from build123d import *

# Parameters (mm, degrees)
F1_DEPTH = 63.5
F0_W     = 25.4
F0_H     = 4.7498
F0_H_2   = 4.7752
F2_DEPTH = 7.9375


with BuildPart() as f1:
    # F0 (on Front) → F1 (new body, symmetric)
    with BuildSketch(Plane.XZ):
        Polygon((25.4, 9.525), (-44.45, 9.525), (-44.45, -9.525), (44.45, -9.525), (44.45, 9.525), align=None)
    extrude(amount=F1_DEPTH, both=True)

    # F0 (on Front) → F2 (join, symmetric)
    with BuildSketch(Plane.XZ):
        with BuildLine():
            add(Edge.make_bspline(
                [(-44.45, 9.525), (-42.0019178226, 33.4759426415), (20.3692746454, 60.014643523), (58.4090455621, 61.8969537879)],
                knots=[0, 0, 0, 0, 115.3620955336, 115.3620955336, 115.3620955336, 115.3620955336], degree=3))
            Line((-44.45, 9.525), (25.4, 9.525))
            Line((25.4, 9.525), (25.4, 27.0245471661))
            ThreePointArc((25.4, 27.0245471661), (34.9609473492, 51.0333051125), (58.4090455621, 61.8969537879))
        make_face()
        Polygon((114.3, 66.675), (114.3, 61.9252), (114.3, 52.3875), (114.3, 42.8752), (114.3, 38.1), (139.7, 38.1), (139.7, 66.675), align=None)
        Polygon((114.3, 61.9252), (88.9, 61.9252), (88.9, 42.8752), (114.3, 42.8752), (114.3, 52.3875), align=None)
        with Locations((101.6, 64.3001)):
            Rectangle(F0_W, F0_H)
        with Locations((101.6, 40.4876)):
            Rectangle(F0_W, F0_H_2)
        with BuildLine():
            Line((25.4, 27.0245471661), (25.4, 9.525))
            Line((25.4, 9.525), (44.45, 9.525))
            Line((44.45, 9.525), (44.45, 27.0245471661))
            ThreePointArc((44.45, 27.0245471661), (48.793134536, 37.9347123308), (59.446120179, 42.8752))
            Line((59.446120179, 42.8752), (88.9, 42.8752))
            Line((88.9, 42.8752), (88.9, 61.9252))
            Line((88.9, 61.9252), (59.0211377493, 61.9252))
            add(Edge.make_bspline(
                [(58.4090455621, 61.8969537879), (58.6137855205, 61.9070848721), (58.8178206284, 61.9165016921), (59.0211377493, 61.9252)],
                knots=[115.3620955336, 115.3620955336, 115.3620955336, 115.3620955336, 115.9830043893, 115.9830043893, 115.9830043893, 115.9830043893], degree=3))
            ThreePointArc((58.4090455621, 61.8969537879), (34.9609473492, 51.0333051125), (25.4, 27.0245471661))
        make_face()
    extrude(amount=F2_DEPTH, both=True)


solid = f1.part
The listing builds one solid part. Answer for the finished solid, in the listing's coordinates (mm). A direction names the side the tool comes from. Give positions to 0.01 mm unless a question says otherwise; leave off trailing zeros. Order: outer loops, then holes, each group sorted by start corner. A loop starts at its lowest first (then second) coordinate and runs counter-clockwise, first axis right, second up. Notation, with made-up numbers: (45, 71.5) - (67, 71.5) arc R19 ccw to (67, 77.5) - close; hole circle Ø6 at (35.25, 35.25). An arc over 180 degrees is marked (long way). Use one line per item in the form item = value.
1) Find section A-A on x = 101. Determine the outline of the cut face in (y, z) (1 decimal).
Verdict:
outline = (-7.9, 38.1) - (7.9, 38.1) - (7.9, 66.7) - (-7.9, 66.7) - close
2) The mould has two halves that part along X. Classify faces 5 (the flat face through (88.9, 0, 41)), 6 (the flat face through (49, -7.938, 39)), 7 (the flat face through (-44.45, -1, 0)): released by +X, released by -X, zero draft, split by the parting line, or undercut.
Verdict:
face_5 = undercut
face_6 = zero draft
face_7 = released by -X
3) Each of these flat-tipped pins is pushed along its axis until it touches: pin 1 (8 mm diameter, centred on x = 68, y = -1, fed in from +Z); pin 2 (18.5 mm diameter, centred on y = 24.5, z = 14, fed in from +X); pin 3 (1.4 mm diameter, centred on y = 2.5, z = 65, fed in from -X). Where does it stop, or does it pass through?
Verdict:
pin_1 = 61.93
pin_2 = 44.45
pin_3 = 88.9
4) Find section B-B on z = 7. Determine the outline of the cut face in (x, y).
Verdict:
outline = (-44.45, -63.5) - (44.45, -63.5) - (44.45, 63.5) - (-44.45, 63.5) - close
5) For faces 1 (the flat face through (74, 0, 42.875)), 2 (the flat face through (49, 7.938, 39)), 3 (the flat face through (88.9, 0, 64)), 4 (the flat face through (114, 0, 38.1)), determine the directions among +Z, -Z, +X, -X, +Y, -Y from which every point of the face is accessible in a straight line to the end or side of a thin tool.
Verdict:
face_1 = -Z, +Y, -Y
face_2 = +Z, +X, -X, +Y
face_3 = +Z, -X, +Y, -Y
face_4 = -Z, +X, +Y, -Y
6) Consider probe 1 along Y at (x, z) = (102, 53); probe 2 along X at (y, z) = (-30, 4); probe 3 along Z at (x, y) = (10, 44) (3 decimals). Determine where each line is inside the solid, lowest interval first. Write a range as [from, to].
Verdict:
probe_1 = [-7.94, 7.94]
probe_2 = [-44.45, 44.45]
probe_3 = [-9.525, 9.525]
